from build123d import *

# Parameters (mm, degrees)
CROQUIS1_R              = 1.5
CROQUIS1_R_2            = 4
SALIENTE_EXTRUIR1_DEPTH = 6
CROQUIS4_R              = 4
SALIENTE_EXTRUIR3_DEPTH = 6
CORTAR_EXTRUIR1_DEPTH   = 6
REDONDEO3_R             = 4
CORTAR_EXTRUIR2_DEPTH   = 6
REDONDEO4_R             = 2.5
REDONDEO6_R             = 10
CORTAR_EXTRUIR3_START   = -6
CROQUIS9_R              = 4
CORTAR_EXTRUIR3_DEPTH   = 6
CROQUIS15_R             = 4
SALIENTE_EXTRUIR4_DEPTH = 6
REDONDEO12_R            = 10
REDONDEO13_R            = 3


with BuildPart() as part:
    # Croquis1 → Saliente-Extruir1 (new body)
    with BuildSketch(Plane.XY):
        with BuildLine():
            Line((-17.112213819, 2.294275414), (-30.516043414, 23.123582692))
            ThreePointArc((-30.516043414, 23.123582692), (-31.14080226, 23.989156666), (-31.854269143, 24.783201331))
            Line((-31.854269143, 24.783201331), (-45.961940777, 38.890872965))
            Line((-45.961940777, 38.890872965), (-106.773123959, 99.702056147))
            Line((-106.773123959, 99.702056147), (-99.702056147, 106.773123959))
            Line((-99.702056147, 106.773123959), (-38.890872965, 45.961940777))
            Line((-38.890872965, 45.961940777), (-24.783201331, 31.854269143))
            ThreePointArc((-24.783201331, 31.854269143), (-23.989156666, 31.14080226), (-23.123582692, 30.516043414))
            Line((-23.123582692, 30.516043414), (-2.294275414, 17.112213819))
            ThreePointArc((-2.294275414, 17.112213819), (-0.610887166, 15.302496804), (0, 12.907567049))
            Line((0, 12.907567049), (0, 7.055686841))
            ThreePointArc((0, 7.055686841), (-0.823113423, 5.438609853), (-2.614937985, 5.15257064))
            Line((-2.614937985, 5.15257064), (-4.503911831, 5.762938925))
            ThreePointArc((-4.503911831, 5.762938925), (-5.518487605, 5.518487605), (-5.762938925, 4.503911831))
            Line((-5.762938925, 4.503911831), (-5.15257064, 2.614937985))
            ThreePointArc((-5.15257064, 2.614937985), (-5.438609853, 0.823113423), (-7.055686841, 0))
            Line((-7.055686841, 0), (-12.907567049, 0))
            ThreePointArc((-12.907567049, 0), (-15.302496804, 0.610887166), (-17.112213819, 2.294275414))
        make_face()
        with Locations((-38.890872965, 38.890872965)):
            Circle(CROQUIS1_R, mode=Mode.SUBTRACT)
        with Locations((-24.04163056, 24.04163056)):
            Circle(CROQUIS1_R, mode=Mode.SUBTRACT)
        with Locations((-15.25, 15.25)):
            Circle(CROQUIS1_R_2, mode=Mode.SUBTRACT)
    extrude(amount=SALIENTE_EXTRUIR1_DEPTH)

    # Croquis4 → Saliente-Extruir3 (add)
    with BuildSketch(Plane.XY.offset(6)):
        Polygon((-106.773123959, 99.702056147), (-118.086832458, 99.702056147), (-132.228968082, 113.844191771), (-132.228968082, 132.228968082), (-113.844191771, 132.228968082), (-99.702056147, 118.086832458), (-99.702056147, 106.773123959), align=None)
        with Locations((-116.672618896, 116.672618896)):
            Circle(CROQUIS4_R, mode=Mode.SUBTRACT)
    extrude(amount=-SALIENTE_EXTRUIR3_DEPTH)

    # Croquis5 → Cortar-Extruir1 (cut)
    with BuildSketch(Plane.XY.offset(6)):
        with BuildLine():
            Line((-127.632774004, 124.450793489), (-125.511453661, 122.329473145))
            ThreePointArc((-125.511453661, 122.329473145), (-122.329473145, 122.329473145), (-122.329473145, 125.511453661))
            Line((-122.329473145, 125.511453661), (-124.450793489, 127.632774004))
            ThreePointArc((-124.450793489, 127.632774004), (-127.632774004, 127.632774004), (-127.632774004, 124.450793489))
        make_face()
        with BuildLine():
            Line((-118.172618896, 108.922618896), (-118.172618896, 106.922618896))
            ThreePointArc((-118.172618896, 106.922618896), (-116.672618896, 105.422618896), (-115.172618896, 106.922618896))
            Line((-115.172618896, 106.922618896), (-115.172618896, 108.922618896))
            ThreePointArc((-115.172618896, 108.922618896), (-116.672618896, 110.422618896), (-118.172618896, 108.922618896))
        make_face()
        with BuildLine():
            Line((-108.922618896, 115.172618896), (-106.922618896, 115.172618896))
            ThreePointArc((-106.922618896, 115.172618896), (-105.422618896, 116.672618896), (-106.922618896, 118.172618896))
            Line((-106.922618896, 118.172618896), (-108.922618896, 118.172618896))
            ThreePointArc((-108.922618896, 118.172618896), (-110.422618896, 116.672618896), (-108.922618896, 115.172618896))
        make_face()
        with BuildLine():
            Line((-124.422618896, 118.172618896), (-126.422618896, 118.172618896))
            ThreePointArc((-126.422618896, 118.172618896), (-127.922618896, 116.672618896), (-126.422618896, 115.172618896))
            Line((-126.422618896, 115.172618896), (-124.422618896, 115.172618896))
            ThreePointArc((-124.422618896, 115.172618896), (-122.922618896, 116.672618896), (-124.422618896, 118.172618896))
        make_face()
        with BuildLine():
            Line((-115.172618896, 124.422618896), (-115.172618896, 126.422618896))
            ThreePointArc((-115.172618896, 126.422618896), (-116.672618896, 127.922618896), (-118.172618896, 126.422618896))
            Line((-118.172618896, 126.422618896), (-118.172618896, 124.422618896))
            ThreePointArc((-118.172618896, 124.422618896), (-116.672618896, 122.922618896), (-115.172618896, 124.422618896))
        make_face()
    extrude(amount=-CORTAR_EXTRUIR1_DEPTH, mode=Mode.SUBTRACT)

    # Redondeo3
    redondeo3_edges = [part.edges().sort_by_distance(p)[0] for p in [
        (-132.228968082, 132.228968082, 3),
    ]]
    fillet(redondeo3_edges, radius=REDONDEO3_R)

    # Croquis7 → Cortar-Extruir2 (cut)
    with BuildSketch(Plane.XY.offset(6)):
        with BuildLine():
            Line((-132.228968082, 113.844191771), (-118.086832458, 99.702056147))
            ThreePointArc((-118.086832458, 99.702056147), (-123.944696834, 107.986327395), (-132.228968082, 113.844191771))
        make_face()
        with BuildLine():
            Line((-113.844191771, 132.228968082), (-99.702056147, 118.086832458))
            ThreePointArc((-99.702056147, 118.086832458), (-107.986327395, 123.944696834), (-113.844191771, 132.228968082))
        make_face()
    extrude(amount=-CORTAR_EXTRUIR2_DEPTH, mode=Mode.SUBTRACT)

    # Redondeo4
    redondeo4_edges = [part.edges().sort_by_distance(p)[0] for p in [
        (-118.086832458, 99.702056147, 3),
        (-132.228968082, 113.844191771, 3),
        (-113.844191771, 132.228968082, 3),
        (-99.702056147, 118.086832458, 3),
    ]]
    fillet(redondeo4_edges, radius=REDONDEO4_R)

    # Redondeo6
    redondeo6_edges = [part.edges().sort_by_distance(p)[0] for p in [
        (-106.773123959, 99.702056147, 3),
        (-99.702056147, 106.773123959, 3),
    ]]
    fillet(redondeo6_edges, radius=REDONDEO6_R)

    # Croquis9 → Cortar-Extruir3 (cut)
    with BuildSketch(Plane.XY.offset(6).offset(CORTAR_EXTRUIR3_START)):
        with BuildLine():
            Line((-23.047623594, 15.976555782), (-31.854269143, 24.783201331))
            ThreePointArc((-31.854269143, 24.783201331), (-31.14080226, 23.989156666), (-30.516043414, 23.123582692))
            Line((-30.516043414, 23.123582692), (-17.112213819, 2.294275414))
            ThreePointArc((-17.112213819, 2.294275414), (-15.302496804, 0.610887166), (-12.907567049, 0))
            Line((-12.907567049, 0), (-7.055686841, 0))
            ThreePointArc((-7.055686841, 0), (-5.438609853, 0.823113423), (-5.15257064, 2.614937985))
            Line((-5.15257064, 2.614937985), (-5.762938925, 4.503911831))
            ThreePointArc((-5.762938925, 4.503911831), (-5.518487605, 5.518487605), (-4.503911831, 5.762938925))
            Line((-4.503911831, 5.762938925), (-2.614937985, 5.15257064))
            ThreePointArc((-2.614937985, 5.15257064), (-0.823113423, 5.438609853), (0, 7.055686841))
            Line((0, 7.055686841), (0, 12.907567049))
            ThreePointArc((0, 12.907567049), (-0.610887166, 15.302496804), (-2.294275414, 17.112213819))
            Line((-2.294275414, 17.112213819), (-23.123582692, 30.516043414))
            ThreePointArc((-23.123582692, 30.516043414), (-23.989156666, 31.14080226), (-24.783201331, 31.854269143))
            Line((-24.783201331, 31.854269143), (-15.976555782, 23.047623594))
            Line((-15.976555782, 23.047623594), (-23.047623594, 15.976555782))
        make_face()
        with Locations((-15.25, 15.25)):
            Circle(CROQUIS9_R, mode=Mode.SUBTRACT)
    extrude(amount=CORTAR_EXTRUIR3_DEPTH, mode=Mode.SUBTRACT)

    # Croquis15 → Saliente-Extruir4 (add)
    with BuildSketch(Plane.XY.offset(6)):
        with BuildLine():
            Line((-19.512089688, 26.5831575), (-15.976555782, 23.047623594))
            Line((-15.976555782, 23.047623594), (-23.047623594, 15.976555782))
            Line((-23.047623594, 15.976555782), (-8.609865422, 1.53879761))
            Line((-8.609865422, 1.53879761), (-4.93762751, 1.898269736))
            ThreePointArc((-4.93762751, 1.898269736), (-3.171999371, 2.840663892), (-2.589885038, 4.755524821))
            Line((-2.589885038, 4.755524821), (-3.381380182, 6.576048667))
            ThreePointArc((-3.381380182, 6.576048667), (-3.236935195, 7.609613418), (-2.251001031, 7.95174537))
            Line((-2.251001031, 7.95174537), (-0.311548805, 7.528310963))
            ThreePointArc((-0.311548805, 7.528310963), (1.454079334, 8.470705119), (2.036193666, 10.385566048))
            Line((2.036193666, 10.385566048), (1.676721541, 14.05780396))
            Line((1.676721541, 14.05780396), (-11.059892894, 23.047623594))
            Line((-11.059892894, 23.047623594), (-19.512089688, 26.5831575))
        make_face()
        with Locations((-13.881053208, 16.502885084)):
            Circle(CROQUIS15_R, mode=Mode.SUBTRACT)
    extrude(amount=-SALIENTE_EXTRUIR4_DEPTH)

    # Redondeo12
    redondeo12_edges = [part.edges().sort_by_distance(p)[0] for p in [
        (-19.512089688, 26.5831575, 3),
        (-11.059892894, 23.047623594, 3),
    ]]
    fillet(redondeo12_edges, radius=REDONDEO12_R)

    # Redondeo13
    redondeo13_edges = [part.edges().sort_by_distance(p)[0] for p in [
        (-8.609865422, 1.53879761, 3),
        (1.676721541, 14.05780396, 3),
    ]]
    fillet(redondeo13_edges, radius=REDONDEO13_R)


solid = part.part
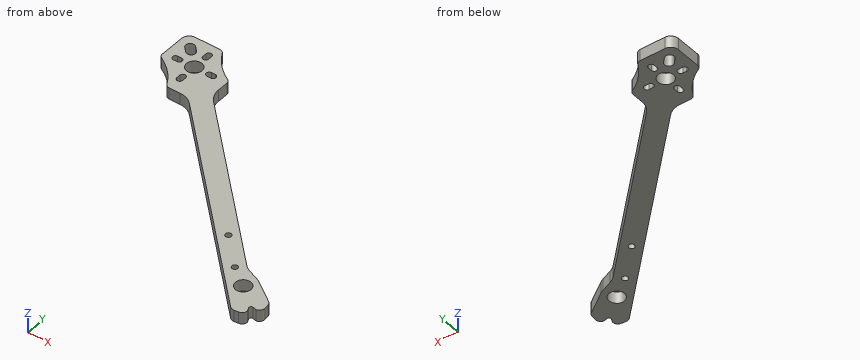
The listing builds one solid part. Answer for the finished solid, in the listing's coordinates (mm). Give positions to 0.01 mm unless a question says otherwise; leave off trailing zeros. Order: outer loops, then holes, each group sorted by start corner. A loop starts at its lowest first (then second) coordinate and runs counter-clockwise, first axis right, second up. Notation, with made-up numbers: (-13.5, -36.5) - (26.5, -36.5) arc R23 ccw to (26.5, -17.5) - close; hole circle Ø6 at (70.25, -10.75). An arc over 180 degrees is marked (long way). Use one line per item in the form item = value.
1) Find section B-B on y = 60.5. Determine the outline of the cut face in (x, z), and give its area (3 significant figures).
Verdict:
outline = (-67.57, 0) - (-53.43, 0) - (-53.43, 6) - (-67.57, 6) - close
area = 84.9 mm^2
2) Each of these flat-tipped pins is pushed along its axis until it touches: pin 1 (2.5 mm diameter, centred on x = -38.89, y = 38.89, fed in from +Z); pin 2 (1 mm diameter, centred on x = -108, z = 3, fed in from -Y); pin 3 (1 mm diameter, centred on y = 107.5, z = 2.5, fed in from -X); pin 4 (2 mm diameter, centred on y = 107.5, z = 3.5, fed in from +X). Where does it stop, or does it pass through?
Verdict:
pin_1 = through
pin_2 = 99.1
pin_3 = -123.96
pin_4 = -98.67
3) Find section C-C on z = 3.15. Give the number of separate pieces and of enclosed holes in the cut face, and give its area (3 significant figures).
Verdict:
separate_pieces = 1
enclosed_holes = 9
area = 2,100 mm^2
4) Find section D-D on x = -84. Determine the outline of the cut face in (y, z).
Verdict:
outline = (76.93, 0) - (91.07, 0) - (91.07, 6) - (76.93, 6) - close
5) Find section A-A on x = -15.5. Determine the outline of the cut face in (y, z), and give its area (3 significant figures).
Verdict:
outline = (8.43, 0) - (12.85, 0) - (12.85, 6) - (8.43, 6) - close; (20.16, 0) - (24.9, 0) - (24.9, 6) - (20.16, 6) - close
area = 55.0 mm^2
6) Consider probe 1 along Y at (x, z) = (-118, 0.9); probe 2 along X at (y, z) = (124, 2.85); probe 3 along X at (y, z) = (125.5, 5.75). Determine where each line is inside the solid, lowest interval first. Write a range as [from, to].
Verdict:
probe_1 = [100.16, 106.22], [109.62, 112.9], [120.45, 123.72], [127.12, 132.23]
probe_2 = [-132.23, -127.18], [-121.67, -118.11], [-115.23, -108.04]
probe_3 = [-132.23, -128.23], [-122.32, -118.17], [-115.17, -109.44]
